Model file for the job. Use its own axes, mm. Face numbers are marked on the shaded views. A direction names the side the tool comes from. Coordinates: 2 decimals unless noted, no trailing zeros. Write each loop counter-clockwise with the first axis right and the second up, starting at its lowest first coordinate (ties: lowest second). Pieces come first, ordered by that corner, then holes. Notation, with made-up numbers: M 13,24.25 L 61,24.25 A13 ccw 61,35.25 Z; hole C 76.5,4.5 d5. An arc over 180 degrees is marked long. Put each result on its own line as item: value. Start each with the question number.
Q1. Cut at A-A (y = 0). Write the cut outline in (x, z).
Q2. Drill centre lines: line 1 along Y through (x, z) = (-0.8, 0); line 2 along Y through (x, z) = (3.5, 4.75); line 3 along Z through (x, y) = (1.75, -2). Where is each one in solid material? Low to high.
Q3. Drop flat-ended pins along their axis: pin 1 (6 mm diameter, centred on y = 0, z = 0, fed in from -X); pin 2 (3 mm diameter, centred on x = 1.5, y = 4.5, fed in from -Z). Give the stop position or say it passes through.
Q4. Which spindle directions (+Z, -Z, +X, -X, +Y, -Y) get a long thin tool onto all of the face, cutting with end or side? Do the marked faces 4 and 5. Say none if no direction does.
Q5. Cut at C-C (x = -0.75). Write the cut outline in (y, z).
Q6. Pull direction Y, two halves, no side cores. Call the marked faces 1, 2 and 3: pulls with the +Y half, pulls with the -Y half, needs draft (parallel to the pull), parting line crosses it, or undercut.
Q7. Cut at D-D (x = 1.5). Write the cut outline in (y, z), then the cut area to 3 significant figures.
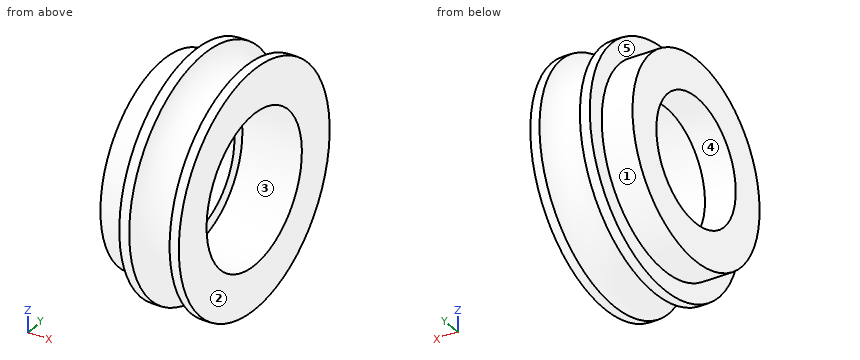
```python
from build123d import *

# Parameters (mm, degrees)
SKETCH_2_R          = 8.712878419
CUT_EXTRUDE_1_DEPTH = 0.7


with BuildPart() as part:
    # 草图1 → 旋转1 (revolve)
    with BuildSketch(Plane.XY, mode=Mode.PRIVATE) as revolve_1_sk:
        with BuildLine():
            Line((0, -9.5), (0.8, -9.5))
            ThreePointArc((0.8, -9.5), (2.430127754, -7.869872246), (4.060255508, -9.5))
            Line((4.060255508, -9.5), (4.8, -9.5))
            Line((4.8, -9.5), (4.8, -6))
            Line((4.8, -6), (0, -6))
            Line((0, -6), (0, -5))
            Line((0, -5), (-3.185969682, -5))
            Line((-3.185969682, -5), (-3.185969682, -8))
            Line((-3.185969682, -8), (0, -8))
            Line((0, -8), (0, -9.5))
        make_face()
    revolve(revolve_1_sk.sketch.rotate(Axis((-3.185969682, 0, 0), (1, 0, 0)), 270), axis=Axis((-3.185969682, 0, 0), (1, 0, 0)))

    # 草图2 → 切除-拉伸1 (cut)
    with BuildSketch(Plane.ZY.offset(3.185969682)):
        Circle(SKETCH_2_R)
    extrude(amount=-CUT_EXTRUDE_1_DEPTH, mode=Mode.SUBTRACT)


solid = part.part
```
Computed values:
1. outline: M -2.49,-8 L 0,-8 L 0,-9.5 L 0.8,-9.5 A1.63 cw 4.06,-9.5 L 4.8,-9.5 L 4.8,-6 L 0,-6 L 0,-5 L -2.49,-5 Z; M -2.49,5 L 0,5 L 0,6 L 4.8,6 L 4.8,9.5 L 4.06,9.5 A1.63 cw 0.8,9.5 L 0,9.5 L 0,8 L -2.49,8 Z
2. line 1: -8 to -5, 5 to 8
2. line 2: -6.77 to -3.67, 3.67 to 6.77
2. line 3: -7.77 to -5.66, 5.66 to 7.77
3. pin 1: through
3. pin 2: z = -8.95
4. face 4: +X, -X
4. face 5: -X
5. outline: C 0,0 d16; hole C 0,0 d10
6. face 1: parting line crosses it
6. face 2: needs draft
6. face 3: undercut
7. outline: C 0,0 d16.32; hole C 0,0 d12
7. area: 96.2 mm2
